For this review, take the finished solid that the model builds, in its own axes (mm). Face numbers are marked on the shaded views. Round coordinates to 2 decimals unless told otherwise and drop trailing zeros. Loops run counter-clockwise (first coordinate to the right, second up) from the corner with the lowest first, then second, coordinate; pieces in that order, holes last.
1. Clearance check with flat-ended pins moving along their axes: pin 1 Ø1.3 at (x, z) = (-1, 6) entering from -Y; pin 2 Ø2 at (y, z) = (3, 12.5) entering from +X; pin 3 Ø4 at (x, z) = (2.5, 7) entering from +Y; pin 4 Ø3.5 at (x, y) = (0, 0) entering from -Z. State where each tip first meets the part, or that it passes through.
2. Consider section C-C on y = -5. State the section outline as (x, z) points, then the cut area to 3 significant figures.
3. Consider section D-D on y = 3.25. State the section outline as (x, z) points, then the cut area to 3 significant figures.
4. To check wall thickness, follow line 1 along Y through (x, z) = (0, 14.75); line 2 along Y through (x, z) = (0, 13.75); line 3 along Z through (x, y) = (-4.5, -3.5). State the ranges of each line that lie inside material, in increasing order.
5. Consider section B-B on z = 4. State the section outline as (x, y) points, then the cut area to 3 significant figures.
6. Draft analysis for pull direction X (two halves, no side actions). For the marked faces 1, 2 and 3, state which applies: released by +X, released by -X, zero draft, split by the parting line, or undercut.
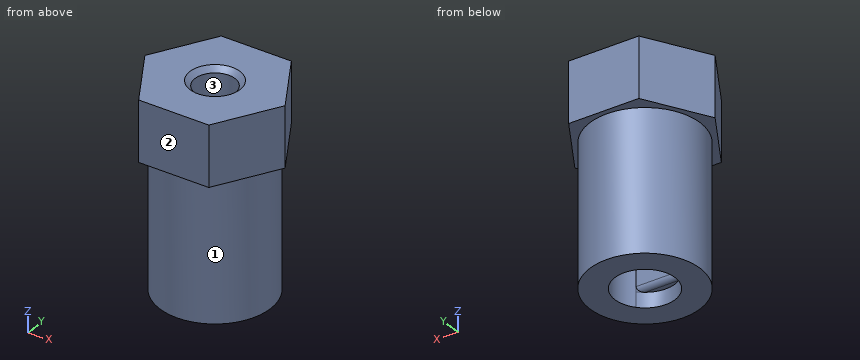
from build123d import *
from build123d.topology import SkipClean

# Parameters (mm, degrees)
SKETCH1_R           = 5.5
BOSS_EXTRUDE1_DEPTH = 14
BOSS_EXTRUDE2_DEPTH = 6
SKETCH3_R           = 1.99
CUT_EXTRUDE1_DEPTH  = 8
CUT_EXTRUDE2_DEPTH  = 12
SKETCH5_R           = 3
CUT_EXTRUDE3_DEPTH  = 1.5
FILLET2_R           = 0.5
CHAMFER1_SIZE       = 0.5


with BuildPart() as part:
    # Sketch1 → Boss-Extrude1 (new body)
    with BuildSketch(Plane.XY):
        Circle(SKETCH1_R)
    extrude(amount=BOSS_EXTRUDE1_DEPTH)

    # Sketch2 → Boss-Extrude2 (add)
    with BuildSketch(Plane.XY.offset(14)):
        Polygon((-6.928203, 0), (-3.464102, -6), (3.464102, -6), (6.928203, 0), (3.464102, 6), (-3.464102, 6), align=None)
    extrude(amount=BOSS_EXTRUDE2_DEPTH)

    # Sketch3 → Cut-Extrude1 (cut)
    with BuildSketch(Plane.XY.offset(20)):
        Circle(SKETCH3_R)
    extrude(amount=-CUT_EXTRUDE1_DEPTH, mode=Mode.SUBTRACT)

    # Sketch4 → Cut-Extrude2 (cut)
    with BuildSketch(Plane(origin=(0, 0, 0), x_dir=(-1, 0, 0), z_dir=(0, 0, -1))):
        with BuildLine():
            Line((-2.236068, 2), (2.236068, 2))
            ThreePointArc((2.236068, 2), (3, 0), (2.236068, -2))
            Line((2.236068, -2), (-2.236068, -2))
            ThreePointArc((-2.236068, -2), (-3, 0), (-2.236068, 2))
        make_face()
    extrude(amount=-CUT_EXTRUDE2_DEPTH, mode=Mode.SUBTRACT)

    # Sketch5 → Cut-Extrude3 (cut)
    with SkipClean():  # the faces are left unmerged after this step: merging them gives an invalid solid
        with BuildSketch(Plane(origin=(0, 0, 0), x_dir=(-1, 0, 0), z_dir=(0, 0, -1))):
            Circle(SKETCH5_R)
        extrude(amount=-CUT_EXTRUDE3_DEPTH, mode=Mode.SUBTRACT)

    # Fillet2
    # the kernel refuses this fillet: 0.5 mm, written as the material it takes off along each edge
    with BuildSketch(Plane(origin=(3.486068, -2, 1.5), x_dir=(0, 0, 1), z_dir=(-1, 0, 0))) as fillet2_piece_1_section:
        with BuildLine():
            CenterArc((FILLET2_R, -FILLET2_R), FILLET2_R, 90, 90)
            Line((0, -FILLET2_R), (0, 0))
            Line((0, 0), (FILLET2_R, 0))
        make_face()
    fillet2_piece_1 = extrude(amount=6.972136, mode=Mode.PRIVATE)
    fillet2_piece_1 = fillet2_piece_1 & Plane(origin=(0, 0, 1.616535), x_dir=(-1, 0, 0), z_dir=(0, 0, -1)) * Cylinder(3, 16, mode=Mode.PRIVATE)
    add(fillet2_piece_1, mode=Mode.SUBTRACT)
    with BuildSketch(Plane(origin=(-3.486068, 2, 1.5), x_dir=(0, 0, 1), z_dir=(1, 0, 0))) as fillet2_piece_2_section:
        with BuildLine():
            CenterArc((FILLET2_R, -FILLET2_R), FILLET2_R, 90, 90)
            Line((0, -FILLET2_R), (0, 0))
            Line((0, 0), (FILLET2_R, 0))
        make_face()
    fillet2_piece_2 = extrude(amount=6.972136, mode=Mode.PRIVATE)
    fillet2_piece_2 = fillet2_piece_2 & Plane(origin=(0, 0, 1.616535), x_dir=(-1, 0, 0), z_dir=(0, 0, -1)) * Cylinder(3, 16, mode=Mode.PRIVATE)
    add(fillet2_piece_2, mode=Mode.SUBTRACT)

    # Chamfer1
    chamfer1_edges = [part.edges().sort_by_distance(p)[0] for p in [
        (-1.99, 0, 20),
    ]]
    chamfer(chamfer1_edges, length=CHAMFER1_SIZE)


solid = part.part
Resolved:
1. pin 1: stops at y = -5.49
1. pin 2: stops at x = 5.12
1. pin 3: stops at y = 5.48
1. pin 4: passes through
2. outline: (-4.04, 14) - (-2.29, 14) - (-2.29, 0) - (2.29, 0) - (2.29, 14) - (4.04, 14) - (4.04, 20) - (-4.04, 20) - close
2. area: 113 mm2
3. outline: (-5.05, 14) - (-4.44, 14) - (-4.44, 0) - (4.44, 0) - (4.44, 14) - (5.05, 14) - (5.05, 20) - (-5.05, 20) - close
3. area: 185 mm2
4. line 1: y = -6 to -1.99, 1.99 to 6
4. line 2: y = -5.5 to -1.99, 1.99 to 5.5
4. line 3: z = 14 to 20
5. outline: circle Ø11 at (0, 0); hole (-2.24, -2) - (2.24, -2) arc R3 ccw to (2.24, 2) - (-2.24, 2) arc R3 ccw to start
5. area: 73.0 mm2
6. face 1: split by the parting line
6. face 2: zero draft
6. face 3: undercut
